from build123d import *

# Parameters (mm, degrees)
SKETCH1_W           = 40
SKETCH1_H           = 30
BOSS_EXTRUDE1_DEPTH = 5
SKETCH2_W           = 21
SKETCH2_H           = 21
CUT_EXTRUDE1_DEPTH  = 2
SKETCH3_W           = 14
SKETCH3_H           = 3
CUT_EXTRUDE2_DEPTH  = 3
SKETCH4_R           = 1.5
CUT_EXTRUDE3_DEPTH  = 3
SKETCH5_R           = 1.5
CUT_EXTRUDE4_DEPTH  = 5
FILLET1_R           = 4


with BuildPart() as part:
    # Sketch1 → Boss-Extrude1 (new body)
    with BuildSketch(Plane(origin=(0, 0, 0), x_dir=(1, 0, 0), z_dir=(0, 1, 0))):
        with Locations((20, 15)):
            Rectangle(SKETCH1_W, SKETCH1_H)
    extrude(amount=BOSS_EXTRUDE1_DEPTH)

    # Sketch2 → Cut-Extrude1 (cut)
    with BuildSketch(Plane(origin=(0, 5, 0), x_dir=(1, 0, 0), z_dir=(0, 1, 0))):
        with Locations((20, 15)):
            Rectangle(SKETCH2_W, SKETCH2_H)
    extrude(amount=-CUT_EXTRUDE1_DEPTH, mode=Mode.SUBTRACT)

    # Sketch3 → Cut-Extrude2 (cut)
    with BuildSketch(Plane(origin=(0, 3, 0), x_dir=(1, 0, 0), z_dir=(0, 1, 0))):
        with Locations((20, 7.5)):
            Rectangle(SKETCH3_W, SKETCH3_H)
    extrude(amount=-CUT_EXTRUDE2_DEPTH, mode=Mode.SUBTRACT)

    # Sketch4 → Cut-Extrude3 (cut)
    with BuildSketch(Plane(origin=(0, 3, 0), x_dir=(1, 0, 0), z_dir=(0, 1, 0))):
        with Locations(Location((13.5, 21.5, 0), (0, 0, 270))):
            Circle(SKETCH4_R)
        with Locations(Location((26.5, 21.5, 0), (0, 0, 270))):
            Circle(SKETCH4_R)
    extrude(amount=-CUT_EXTRUDE3_DEPTH, mode=Mode.SUBTRACT)

    # Sketch5 → Cut-Extrude4 (cut)
    with BuildSketch(Plane(origin=(0, 5, 0), x_dir=(1, 0, 0), z_dir=(0, 1, 0))):
        with Locations(Location((5, 25, 0), (0, 0, 90))):
            Circle(SKETCH5_R)
        with Locations(Location((35, 5, 0), (0, 0, 90))):
            Circle(SKETCH5_R)
        with Locations(Location((35, 25, 0), (0, 0, 270))):
            Circle(SKETCH5_R)
        with Locations(Location((5, 5, 0), (0, 0, 270))):
            Circle(SKETCH5_R)
    extrude(amount=-CUT_EXTRUDE4_DEPTH, mode=Mode.SUBTRACT)

    # Fillet1
    fillet1_edges = [part.edges().sort_by_distance(p)[0] for p in [
        (0, 2.5, -30),
        (40, 2.5, -30),
        (40, 2.5, 0),
        (0, 2.5, 0),
    ]]
    fillet(fillet1_edges, radius=FILLET1_R)


solid = part.part
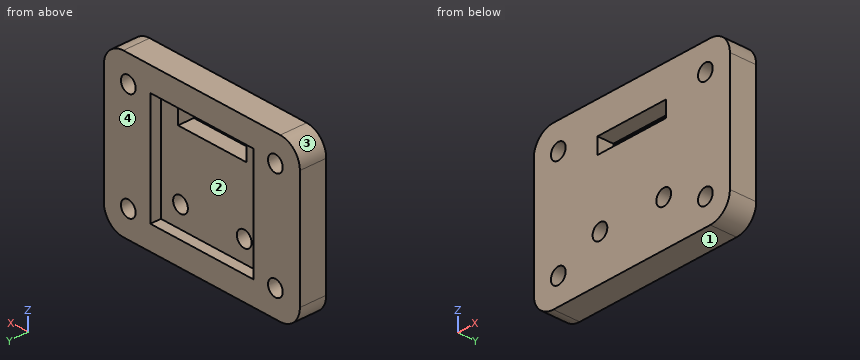
The listing builds one solid part. Answer for the finished solid, in the listing's coordinates (mm). Face numbers are marked on the shaded views. Round coordinates to 2 decimals unless told otherwise and drop trailing zeros. Order: outer loops, then holes, each group sorted by start corner. A loop starts at its lowest first (then second) coordinate and runs counter-clockwise, first axis right, second up. Notation, with made-up numbers: M 52.5,-38.5 L 62.5,-38.5 A31 ccw 62.5,-12.5 Z; hole C 58.5,43.5 d8. An arc over 180 degrees is marked long. Answer in a Markdown table with one row per item. Add a question column.
1) The part is cut by section C-C on y = 2.2. Determine the outline of the cut face in (x, z).
2) Flat-ended cylindrical pins translate along their axes: pin 1 Ø4 at (x, z) = (35, -25) entering from -Y; pin 2 Ø6.5 at (x, z) = (16, -10) entering from +Y. Find the tip coordinate at first contact, or state that the pin passes through.
3) The part is cut by section B-B on x = 35. Determine the outline of the cut face in (y, z).
4) The part is cut by section D-D on z = -18. Determine the outline of the cut face in (x, y).
5) Determine the mould class of the marked faces 1, 2, 3 and 4 for opening direction Z: pulls with the +Z half, pulls with the -Z half, needs draft (parallel to the pull), parting line crosses it, or undercut.
6) The part is cut by section A-A on z = -21.5. Determine the outline of the cut face in (x, y).
7) Consider line 1 along X through (y, z) = (1.7, -25); line 2 along X through (y, z) = (4, -25); line 3 along X through (y, z) = (1.5, -21.5). Determine where each line is inside the solid, lowest interval first. Write a range as from..to.
Findings below:
| question | item | result |
|---|---|---|
| 1 | outline | M 0,-26 A4 ccw 4,-30 L 36,-30 A4 ccw 40,-26 L 40,-4 A4 ccw 36,0 L 4,0 A4 ccw 0,-4 Z; hole C 5,-25 d3; hole C 5,-5 d3; hole C 13.5,-21.5 d3; hole M 13,-9 L 27,-9 L 27,-6 L 13,-6 Z; hole C 26.5,-21.5 d3; hole C 35,-25 d3; hole C 35,-5 d3 |
| 2 | pin 1 | stops at y = 0 |
| 2 | pin 2 | stops at y = 3 |
| 3 | outline | M 0,-30 L 5,-30 L 5,-26.5 L 0,-26.5 Z; M 0,-23.5 L 5,-23.5 L 5,-6.5 L 0,-6.5 Z; M 0,-3.5 L 5,-3.5 L 5,0 L 0,0 Z |
| 4 | outline | M 0,0 L 40,0 L 40,5 L 30.5,5 L 30.5,3 L 9.5,3 L 9.5,5 L 0,5 Z |
| 5 | face 1 | pulls with the -Z half |
| 5 | face 2 | undercut |
| 5 | face 3 | pulls with the +Z half |
| 5 | face 4 | needs draft |
| 6 | outline | M 0,0 L 12,0 L 12,3 L 9.5,3 L 9.5,5 L 0,5 Z; M 15,0 L 25,0 L 25,3 L 15,3 Z; M 28,0 L 40,0 L 40,5 L 30.5,5 L 30.5,3 L 28,3 Z |
| 7 | line 1 | x = 0..3.5, 6.5..33.5, 36.5..40 |
| 7 | line 2 | x = 0..3.5, 6.5..9.5, 30.5..33.5, 36.5..40 |
| 7 | line 3 | x = 0..12, 15..25, 28..40 |
